Can you work these out from the model? Positions are in its coordinate system, mm. A direction names the side the tool comes from. Give positions to 0.01 mm unless a question says otherwise; leave off trailing zeros. Order: outer loops, then holes, each group sorted by start corner. A loop starts at its lowest first (then second) coordinate and runs counter-clockwise, first axis right, second up. Notation, with made-up numbers: M 27.5,31 L 50.5,31 A23 cw 50.5,39 Z; hole C 58.5,62.25 d10. An arc over 180 degrees is marked long. Use one line per item in the form item = value. Start each with the question number.
1. I need wall thicknesses on L1, parallel to Z at x = 1, y = 36.5; L2, parallel to X at y = 18, z = 9; L3, parallel to X at y = -3.5, z = 9.75. Which ranges of each line are inside material? Lowest first, please.
2. Will these pins go through, and if not, where does the flat tip stop? P1, Ø1, axis at x = -16.5, z = 6.5, coming from the -Y side; P2, Ø2, axis at x = 10.5, y = 1, coming from the -Z side.
3. For faces 1 (the face through (-1, -50, 2)), 2 (the face through (-12, 23, 5)), which set-ups out of +Z, -Z, +X, -X, +Y, -Y let a thin tool reach every point of the face, with its end or its side?
4. I want a section at A-A, the plane x = 0. List the corners of the cut face in (y, z) for me.
5. I want a section at C-C, the plane x = 38. List the corners of the cut face in (y, z) for me, and give its area (3 significant figures).
```python
from build123d import *

# Parameters (mm, degrees)
SKETCH_1_W      = 100
SKETCH_1_H      = 100
EXTRUDE_1_DEPTH = 5
SKETCH_2_R      = 22.5
EXTRUDE_2_DEPTH = 5
DRAFT_1_ANGLE   = 15
FILLET_1_R      = 2


with BuildPart() as part:
    # 草图1 → 凸台-拉伸1 (new body)
    with BuildSketch(Plane.XY):
        Rectangle(SKETCH_1_W, SKETCH_1_H)
    extrude(amount=EXTRUDE_1_DEPTH)

    # 草图2 → 凸台-拉伸2 (add)
    with BuildSketch(Plane.XY.offset(5)):
        Circle(SKETCH_2_R)
    extrude(amount=EXTRUDE_2_DEPTH)

    # 拔模1
    draft_1_faces = [part.faces().sort_by_distance(p)[0] for p in [
        (-22.5, 0, 7.5),
    ]]
    draft(draft_1_faces, Plane.XY.offset(10), DRAFT_1_ANGLE)

    # 圆角1
    fillet_1_edges = [part.edges().sort_by_distance(p)[0] for p in [
        (-23.839745962, 0, 5),
        (-22.5, 0, 10),
    ]]
    fillet(fillet_1_edges, radius=FILLET_1_R)


solid = part.part
```
Check result:
q1.L1 = 0 to 5
q1.L2 = -13.83 to 13.83
q1.L3 = -21.65 to 21.65
q2.P1 = -17.18
q2.P2 = 0
q3.face_1 = +Z, -Z, +X, -X, -Y
q3.face_2 = +Z
q4.outline = M -50,0 L 50,0 L 50,5 L 25.37,5 A2 cw 23.44,6.48 L 22.9,8.52 A2 ccw 20.97,10 L -20.97,10 A2 ccw -22.9,8.52 L -23.44,6.48 A2 cw -25.37,5 L -50,5 Z
q5.outline = M -50,0 L 50,0 L 50,5 L -50,5 Z
q5.area = 500 mm2
